Answer from the drawing. Dimensions are ordinates in mm from the lowest x, y and z of the part. Round coordinates to 2 decimals unless told otherwise and drop trailing zeros. Loops run counter-clockwise (first coordinate to the right, second up) from the corner with the lowest first, then second, coordinate; pieces in that order, holes last. Notation, with made-up numbers: M -3.5,8.25 L 50.5,8.25 A25 ccw 50.5,28.25 Z; hole C 24.5,59.5 d5. An arc over 180 degrees is marked long. Answer as a JSON object with one key per item and string values.
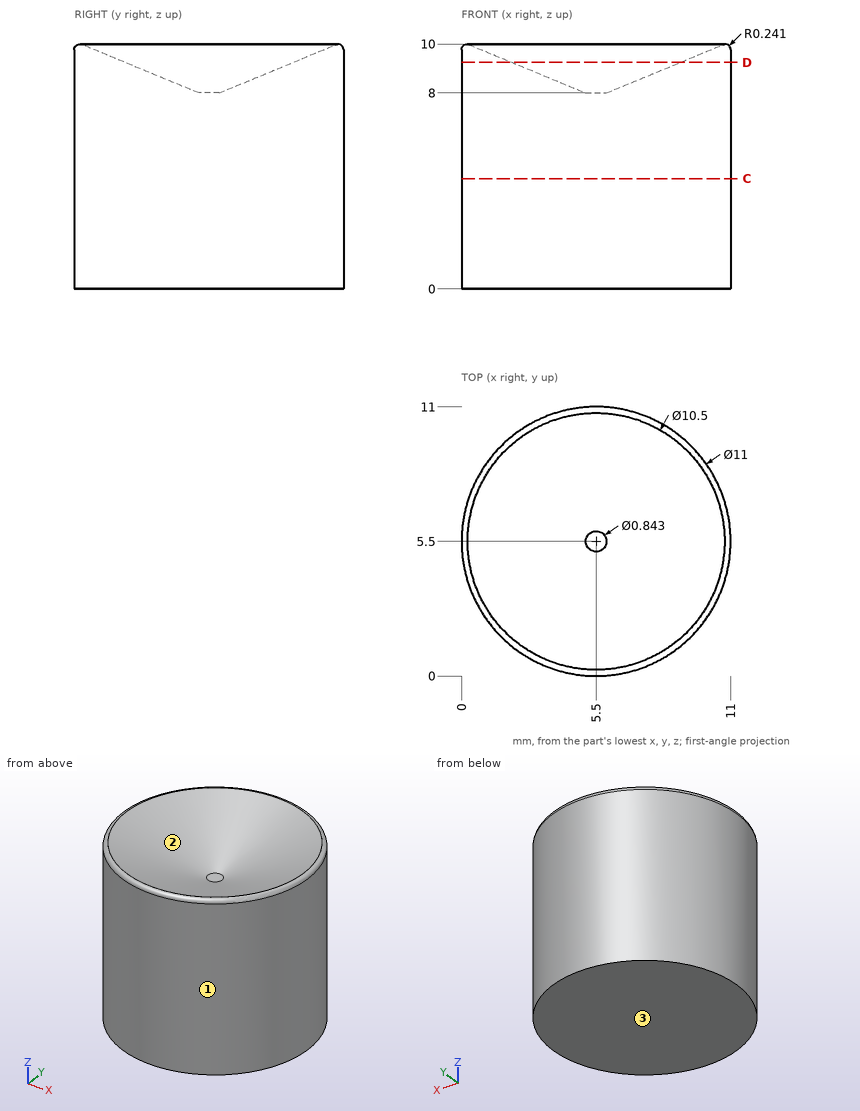
Item 1: Determine the mould class of the marked faces 1, 2 and 3 for opening direction Y: released by +Y, released by -Y, zero draft, split by the parting line, or undercut.
Values follow:
{"face 1": "split by the parting line", "face 2": "undercut", "face 3": "zero draft"}
Item 2: Straight lines are drawn through the part: line 1 (Y direction, x = 5, z = 9.25) (1 decimal); line 2 (Y direction, x = 2, z = 2.25); line 3 (Y direction, x = 4, z = 2). For each, find the intervals that lie inside material, in ascending order.
Values follow:
{"line 1": "0 to 2.1, 8.9 to 11", "line 2": "1.26 to 9.74", "line 3": "0.21 to 10.79"}
Item 3: Flat-ended cylindrical pins translate along their axes: P1, Ø2, axis at x = 8.5, z = 2.5, coming from the -Y side; P2, Ø1.5, axis at x = 8, z = 7, coming from the +Y side (1 decimal); P3, Ø0.7, axis at x = 5.5, y = 5.5, coming from the +Z side. Find the tip coordinate at first contact, or state that the pin passes through.
Values follow:
{"P1": "y = 0.38", "P2": "y = 10.7", "P3": "z = 8"}
Item 4: The part is cut by section D-D (z = 9.25). Give the vertices of the cut face in (x, y).
Values follow:
{"outline": "C 5.5,5.5 d11; hole C 5.5,5.5 d6.88"}
Item 5: The part is cut by section C-C (z = 4.5). Give the vertices of the cut face in (x, y).
Values follow:
{"outline": "C 5.5,5.5 d11"}
